Read the model definition and answer for the solid it produces. Units are mm, in the model's axes. Face numbers are marked on the shaded views. A direction names the side the tool comes from. Give positions to 0.01 mm unless a question says otherwise; leave off trailing zeros. Loops run counter-clockwise (first coordinate to the right, second up) from the corner with the lowest first, then second, coordinate; pieces in that order, holes last. Notation, with made-up numbers: (83, 3) - (126, 3) arc R22 ccw to (126, 35) - close; hole circle Ø10 at (1, 62.5). An arc over 180 degrees is marked (long way). Use a Markdown table: item, result. Add a question column.
Item 1: Which of the six approach directions +Z, -Z, +X, -X, +Y, -Y give full straight-line access (tool end or side, diameter ignored) to the marked faces 1 and 2?
Item 2: Consider probe 1 along Z at (x, y) = (1.75, -2.9); probe 2 along Z at (x, y) = (-3.75, -2.75); probe 3 along X at (y, z) = (-1.9, 0.75). Determine where each line is inside the solid, lowest interval first. Write a range as [from, to].
Item 3: For a pull along Z with two mould halves and no side action, classify the marked faces 3, 4 and 5 as +Z half, -Z half, draft (parallel to the pull), parting line (faces both ways), or undercut.
Item 4: A cutting plane is placed at B-B (z = 0.25). Determine the outline of the cut face in (x, y).
Item 5: A cutting plane is placed at A-A (x = 2.5). Determine the outline of the cut face in (y, z).
Item 6: A cutting plane is placed at C-C (x = -1.5). Determine the outline of the cut face in (y, z).
Item 7: A cutting plane is placed at D-D (y = -2.95). Determine the outline of the cut face in (x, z), plus the area to 3 significant figures.
Item 8: Each of these flat-tipped pins is pushed along its axis until it touches: P1, Ø1.5, axis at x = -3.5, y = -3.5, coming from the +Z side; P2, Ø1, axis at y = -1, z = 2, coming from the +X side. Where does it stop, or does it pass through?
from build123d import *

# Parameters (mm, degrees)
F0_R         = 1.15
F1_DEPTH     = 4
F2_R         = 1.5
F3_DEPTH     = 5
F4_T1_DEPTH  = 9.4903810568
F4_T3_DEPTH  = 1
F4_T5_DEPTH  = 10.75
F4_T7_DEPTH  = 3.2
F4_S11_W     = 1.5
F4_S11_H     = 1.5
F4_T12_DEPTH = 1.5
F4_S17_W     = 1.5
F4_S17_H     = 1.5
F4_T18_DEPTH = 1.5
F4_S23_W     = 1.5
F4_S23_H     = 1.5
F4_T24_DEPTH = 1.5
F4_S29_W     = 1.5
F4_S29_H     = 1.5
F4_T30_DEPTH = 1.5


# Not quite as in the source:
# - a fillet or chamfer that OpenCascade refuses, or shapes differently, is made with other operations: its cross-section is extruded or revolved along the edge and cut away or added


with BuildPart() as f1:
    # F0 (on Front) → F1 (new body)
    with BuildSketch(Plane.XZ):
        with BuildLine():
            Line((5, 3.1), (-3.5, 3.1))
            ThreePointArc((-3.5, 3.1), (-3.9393398282, 2.0393398282), (-5, 1.6))
            Line((-5, 1.6), (-5, -1.6))
            ThreePointArc((-5, -1.6), (-3.9393398282, -2.0393398282), (-3.5, -3.1))
            Line((-3.5, -3.1), (5, -3.1))
            Line((5, -3.1), (5, 3.1))
        make_face()
        with Locations((2.5, 0)):
            Circle(F0_R, mode=Mode.SUBTRACT)
    extrude(amount=F1_DEPTH)

    # F2 (on face) → F3 (cut)
    with BuildSketch(Plane(origin=(-5, 0, 0), x_dir=(0, -1, 0), z_dir=(-1, 0, 0))):
        with Locations((1.9687709864, 0)):
            Circle(F2_R)
    extrude(amount=-F3_DEPTH, mode=Mode.SUBTRACT)

    # F4: fillet of radius 1.5 on 10 edges, made by hand

    # F4_s2 → F4_t1 (cut)
    with BuildSketch(Plane.XZ.offset(-2.7451905284)):
        with BuildLine():
            ThreePointArc((-2.4019237886, 3.1), (-3.1519237886, 2.8990381057), (-3.7009618943, 2.35))
            ThreePointArc((-3.7009618943, 2.35), (-3.5511112606, 2.7117714323), (-3.5, 3.1))
            Line((-3.5, 3.1), (-2.4019237886, 3.1))
        make_face()
        with BuildLine():
            ThreePointArc((-2.4019237886, -3.1), (-3.1519237886, -2.8990381057), (-3.7009618943, -2.35))
            ThreePointArc((-3.7009618943, -2.35), (-3.5511112606, -2.7117714323), (-3.5, -3.1))
            Line((-3.5, -3.1), (-2.4019237886, -3.1))
        make_face()
    extrude(amount=F4_T1_DEPTH, mode=Mode.SUBTRACT)

    # F4_s4 → F4_t3 (cut)
    with BuildSketch(Plane.XZ.offset(1.5)):
        with BuildLine():
            ThreePointArc((3.5, 3.1), (4.5606601718, 2.6606601718), (5, 1.6))
            Line((5, 1.6), (5, 3.1))
            Line((5, 3.1), (3.5, 3.1))
        make_face()
        with BuildLine():
            ThreePointArc((5, -1.6), (4.5606601718, -2.6606601718), (3.5, -3.1))
            Line((3.5, -3.1), (5, -3.1))
            Line((5, -3.1), (5, -1.6))
        make_face()
    extrude(amount=F4_T3_DEPTH, mode=Mode.SUBTRACT)

    # F4_s6 → F4_t5 (cut)
    with BuildSketch(Plane.YZ.offset(-7.25)):
        with BuildLine():
            ThreePointArc((-2.5, 3.1), (-3.5606601718, 2.6606601718), (-4, 1.6))
            Line((-4, 1.6), (-4, 3.1))
            Line((-4, 3.1), (-2.5, 3.1))
        make_face()
        with BuildLine():
            ThreePointArc((-1.5, 3.1), (-0.4393398282, 2.6606601718), (0, 1.6))
            Line((0, 1.6), (0, 3.1))
            Line((0, 3.1), (-1.5, 3.1))
        make_face()
        with BuildLine():
            ThreePointArc((0, -1.6), (-0.4393398282, -2.6606601718), (-1.5, -3.1))
            Line((-1.5, -3.1), (0, -3.1))
            Line((0, -3.1), (0, -1.6))
        make_face()
        with BuildLine():
            ThreePointArc((-4, -1.6), (-3.5606601718, -2.6606601718), (-2.5, -3.1))
            Line((-2.5, -3.1), (-4, -3.1))
            Line((-4, -3.1), (-4, -1.6))
        make_face()
    extrude(amount=F4_T5_DEPTH, mode=Mode.SUBTRACT)

    # F4_s8 → F4_t7 (cut)
    with BuildSketch(Plane.XY.offset(-1.6)):
        with BuildLine():
            ThreePointArc((5, -1.5), (4.5606601718, -0.4393398282), (3.5, 0))
            Line((3.5, 0), (5, 0))
            Line((5, 0), (5, -1.5))
        make_face()
        with BuildLine():
            ThreePointArc((5, -2.5), (4.5606601718, -3.5606601718), (3.5, -4))
            Line((3.5, -4), (5, -4))
            Line((5, -4), (5, -2.5))
        make_face()
    extrude(amount=F4_T7_DEPTH, mode=Mode.SUBTRACT)


with BuildPart() as f4_tool10:
    # F4_s11 → F4_t12 (new body)
    with BuildSketch(Plane.XY.offset(1.6)):
        with Locations((4.25, -0.75)):
            Rectangle(F4_S11_W, F4_S11_H)
    extrude(amount=F4_T12_DEPTH)

    # F4_s13 → F4_t14 (revolve, cut)
    with BuildSketch(Plane(origin=(3.5, -1.5, 1.6), x_dir=(-0.7071067812, -0.7071067812, 0), z_dir=(-0.7071067812, 0.7071067812, 0))):
        with BuildLine():
            ThreePointArc((0, -1.5), (1.5, 0), (0, 1.5))
            Line((0, 1.5), (0, -1.5))
        make_face()
    revolve(axis=Axis((3.5, -1.5, 1.6), (0, 0, 1)), mode=Mode.SUBTRACT)


with BuildPart() as f1_1:
    add(f1.part)

    # F4_t9: cut F4_tool10
    add(f4_tool10.part, mode=Mode.SUBTRACT)


with BuildPart() as f4_tool16:
    # F4_s17 → F4_t18 (new body)
    with BuildSketch(Plane.XY.offset(1.6)):
        with Locations((4.25, -3.25)):
            Rectangle(F4_S17_W, F4_S17_H)
    extrude(amount=F4_T18_DEPTH)

    # F4_s19 → F4_t20 (revolve, cut)
    with BuildSketch(Plane(origin=(3.5, -2.5, 1.6), x_dir=(-0.7071067812, 0.7071067812, 0), z_dir=(0.7071067812, 0.7071067812, 0))):
        with BuildLine():
            ThreePointArc((0, -1.5), (1.5, 0), (0, 1.5))
            Line((0, 1.5), (0, -1.5))
        make_face()
    revolve(axis=Axis((3.5, -2.5, 1.6), (0, 0, 1)), mode=Mode.SUBTRACT)


with BuildPart() as f1_2:
    add(f1_1.part)

    # F4_t15: cut F4_tool16
    add(f4_tool16.part, mode=Mode.SUBTRACT)


with BuildPart() as f4_tool22:
    # F4_s23 → F4_t24 (new body)
    with BuildSketch(Plane.YZ.offset(3.5)):
        with Locations((-0.75, -2.35)):
            Rectangle(F4_S23_W, F4_S23_H)
    extrude(amount=F4_T24_DEPTH)

    # F4_s25 → F4_t26 (revolve, cut)
    with BuildSketch(Plane(origin=(3.5, -1.5, -1.6), x_dir=(0, -0.7071067812, 0.7071067812), z_dir=(0, 0.7071067812, 0.7071067812))):
        with BuildLine():
            ThreePointArc((0, -1.5), (1.5, 0), (0, 1.5))
            Line((0, 1.5), (0, -1.5))
        make_face()
    revolve(axis=Axis((3.5, -1.5, -1.6), (1, 0, 0)), mode=Mode.SUBTRACT)


with BuildPart() as f1_3:
    add(f1_2.part)

    # F4_t21: cut F4_tool22
    add(f4_tool22.part, mode=Mode.SUBTRACT)


with BuildPart() as f4_tool28:
    # F4_s29 → F4_t30 (new body)
    with BuildSketch(Plane.YZ.offset(3.5)):
        with Locations((-3.25, -2.35)):
            Rectangle(F4_S29_W, F4_S29_H)
    extrude(amount=F4_T30_DEPTH)

    # F4_s31 → F4_t32 (revolve, cut)
    with BuildSketch(Plane(origin=(3.5, -2.5, -1.6), x_dir=(0, 0.7071067812, 0.7071067812), z_dir=(0, 0.7071067812, -0.7071067812))):
        with BuildLine():
            ThreePointArc((0, -1.5), (1.5, 0), (0, 1.5))
            Line((0, 1.5), (0, -1.5))
        make_face()
    revolve(axis=Axis((3.5, -2.5, -1.6), (1, 0, 0)), mode=Mode.SUBTRACT)


with BuildPart() as f1_4:
    add(f1_3.part)

    # F4_t27: cut F4_tool28
    add(f4_tool28.part, mode=Mode.SUBTRACT)


solid = f1_4.part
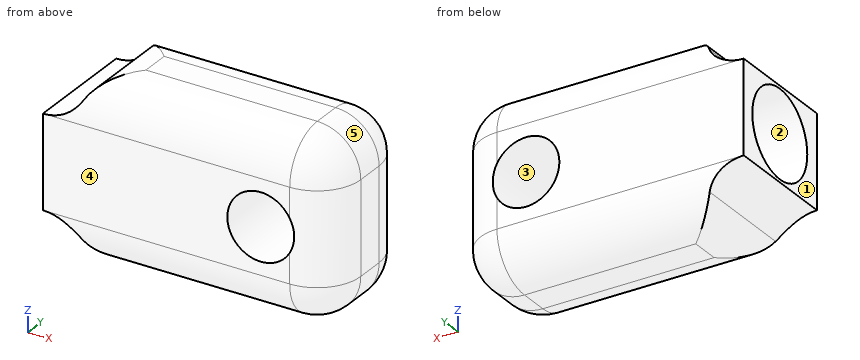
Geometry says:
| question | item | result |
|---|---|---|
| 1 | face 1 | +Z, -Z, -X, +Y, -Y |
| 1 | face 2 | -X |
| 2 | probe 1 | [-3.05, -0.87], [0.87, 3.05] |
| 2 | probe 2 | [-2.27, -1.28], [1.28, 2.27] |
| 2 | probe 3 | [0, 1.63], [3.37, 5] |
| 3 | face 3 | undercut |
| 3 | face 4 | draft |
| 3 | face 5 | +Z half |
| 4 | outline | (-5, -4) - (1.38, -4) - (1.38, 0) - (-5, 0) - (-5, -0.49) - (0, -0.49) - (0, -3.45) - (-5, -3.45) - close; (3.62, -3.99) arc R1.5 ccw to (5, -2.5) - (5, -1.5) arc R1.5 ccw to (3.62, -0.01) - close |
| 5 | outline | (-4, -1.6) arc R1.5 ccw to (-2.5, -3.1) - (-1.5, -3.1) arc R1.5 ccw to (0, -1.6) - (0, -1.15) - (-4, -1.15) - close; (-4, 1.15) - (0, 1.15) - (0, 1.6) arc R1.5 ccw to (-1.5, 3.1) - (-2.5, 3.1) arc R1.5 ccw to (-4, 1.6) - close |
| 6 | outline | (-4, -1.6) arc R1.5 ccw to (-2.5, -3.1) - (-1.5, -3.1) arc R1.5 ccw to (0, -1.6) - (0, 1.6) arc R1.5 ccw to (-1.5, 3.1) - (-2.5, 3.1) arc R1.5 ccw to (-4, 1.6) - close; hole circle Ø3 at (-1.97, 0) |
| 7 | outline | (-5, -1.6) arc R1.5 cw to (-3.7, -2.35) arc R1.5 ccw to (-2.85, -3.03) - (3.5, -3.03) arc R1.43 ccw to (4.93, -1.6) - (4.93, 1.6) arc R1.43 ccw to (3.5, 3.03) - (-2.85, 3.03) arc R1.5 ccw to (-3.7, 2.35) arc R1.5 cw to (-5, 1.6) - (-5, 1.13) - (0, 1.13) - (0, -1.13) - (-5, -1.13) - close; hole circle Ø2.3 at (2.5, 0) |
| 7 | area | 40.2 mm² |
| 8 | P1 | z = 3.01 |
| 8 | P2 | x = 4.99 |
